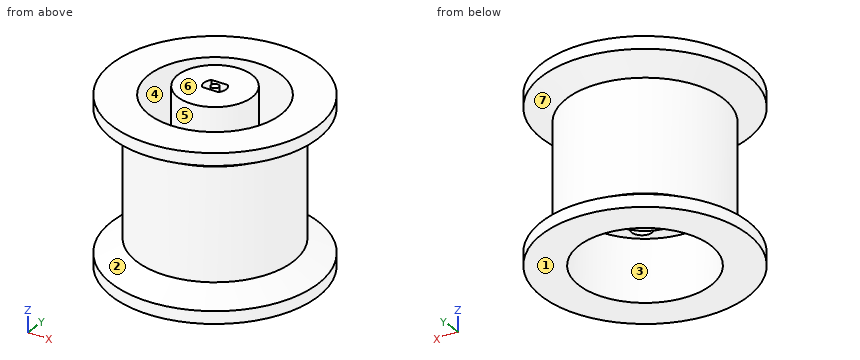
from build123d import *

# Parameters (mm, degrees)
ESQUISSE1_R                  = 25
ESQUISSE1_R_2                = 8
BOSS_EXTRU_1_DEPTH           = 20
ESQUISSE2_R                  = 16
ENL_V_MAT_EXTRU_1_DEPTH      = 15
ESQUISSE3_R                  = 2.5
ENL_V_MAT_EXTRU_2_DEPTH      = 44.301270189
R_P_TITION_CIRCULAIRE1_COUNT = 5
BOSS_EXTRU_2_DEPTH           = 17
BOSS_EXTRU_2_DEPTH_BACK      = 12
ESQUISSE4_R                  = 9
ESQUISSE4_R_2                = 8
BOSS_EXTRU_7_START           = -29
ESQUISSE13_R                 = 8
BOSS_EXTRU_7_DEPTH           = 29
ENL_V_MAT_EXTRU_3_DEPTH      = 7.7
ESQUISSE12_R                 = 0.945
BOSS_EXTRU_6_DEPTH           = 7.7


with BuildPart() as part:
    # Esquisse1 → Boss.-Extru.1 (new, symmetric)
    with BuildSketch(Plane.XY):
        Circle(ESQUISSE1_R)
        Circle(ESQUISSE1_R_2, mode=Mode.SUBTRACT)
    extrude(amount=BOSS_EXTRU_1_DEPTH, both=True)

    # Esquisse2 → Enlèv. mat.-Extru.1 (cut)
    with BuildSketch(Plane.XY.offset(20)):
        Circle(ESQUISSE2_R)
    enl_v_mat_extru_1 = extrude(amount=-ENL_V_MAT_EXTRU_1_DEPTH, mode=Mode.SUBTRACT)

    # Symétrie1: Enlèv. mat.-Extru.1 across plane
    add(enl_v_mat_extru_1.mirror(Plane.XY), mode=Mode.SUBTRACT)

    # Esquisse3 → Enlèv. mat.-Extru.2 (cut, through all)
    with BuildSketch(Plane.XY.offset(5)):
        with Locations((0, 12)):
            Circle(ESQUISSE3_R)
    enl_v_mat_extru_2 = extrude(amount=-ENL_V_MAT_EXTRU_2_DEPTH, mode=Mode.SUBTRACT)

    # Répétition circulaire1: Enlèv. mat.-Extru.2 ×5 about axis
    r_p_tition_circulaire1_axis = Axis((0, 0, 0), (0, 0, 1))
    for i in range(1, R_P_TITION_CIRCULAIRE1_COUNT):
        add(enl_v_mat_extru_2.rotate(r_p_tition_circulaire1_axis, i * 360 / R_P_TITION_CIRCULAIRE1_COUNT), mode=Mode.SUBTRACT)

    # Esquisse4 → Boss.-Extru.2 (add, two sides: drawn at the far end of the back side and taken through both)
    with BuildSketch(Plane.XY.offset(5).offset(-BOSS_EXTRU_2_DEPTH_BACK)):
        Circle(ESQUISSE4_R)
        Circle(ESQUISSE4_R_2, mode=Mode.SUBTRACT)
    extrude(amount=BOSS_EXTRU_2_DEPTH + BOSS_EXTRU_2_DEPTH_BACK)

    # Esquisse5 → Enlèvement de matière-Révolution1 (revolve, cut)
    with BuildSketch(Plane(origin=(0, 0, 0), x_dir=(1, 0, 0), z_dir=(0, 1, 0))):
        Polygon((-25, 17), (-19, 13.535898385), (-19, -13.535898385), (-25, -17), align=None)
    revolve(axis=Axis((0, 0, -25.284593115), (0, 0, 1)), mode=Mode.SUBTRACT)

    # Esquisse13 → Boss.-Extru.7 (add)
    with BuildSketch(Plane.XY.offset(22).offset(BOSS_EXTRU_7_START)):
        Circle(ESQUISSE13_R)
    extrude(amount=BOSS_EXTRU_7_DEPTH)

    # Esquisse11 → Enlèv. mat.-Extru.3 (cut)
    with BuildSketch(Plane.XY.offset(22)):
        with BuildLine():
            Line((-2.015, 1.8), (2.015, 1.8))
            ThreePointArc((2.015, 1.8), (2.695784465, 0), (2.015, -1.8))
            Line((2.015, -1.8), (-2.015, -1.8))
            ThreePointArc((-2.015, -1.8), (-2.695784465, 0), (-2.015, 1.8))
        make_face()
    extrude(amount=-ENL_V_MAT_EXTRU_3_DEPTH, mode=Mode.SUBTRACT)

    # Esquisse12 → Boss.-Extru.6 (add)
    with BuildSketch(Plane.XY.offset(14.3)):
        Circle(ESQUISSE12_R)
    extrude(amount=BOSS_EXTRU_6_DEPTH)


solid = part.part
For this review, take the finished solid that the model builds, in its own axes (mm). Face numbers are marked on the shaded views. A direction names the side the tool comes from. Round coordinates to 2 decimals unless told otherwise and drop trailing zeros. Write each loop counter-clockwise with the first axis right and the second up, starting at its lowest first coordinate (ties: lowest second). Pieces come first, ordered by that corner, then holes. Notation, with made-up numbers: M 49.25,70 L 68.25,70 A17 ccw 68.25,102 Z; hole C 1,37 d3. An arc over 180 degrees is marked long. Write item = value, one per line. Start each with the question number.
(1) For line 1 along Y through (x, z) = (0, 9); line 2 along Y through (x, z) = (0, -9.25); line 3 along Y through (x, z) = (1, -5.5), list the stretches that pass through material, from the lowest coordinate up.
(2) We need section A-A (z = 1.5). Give the boundary of the cut face in (x, y), then the cut area to 3 significant figures.
(3) For the marked faces 5, 6 and 7, list the 3-axis set-ups (+Z, -Z, +X, -X, +Y, -Y) from which the entire face can be reached by the end or side of a thin tool; tool diameter is ignored.
(4) The part is to be moulded in two halves that separate along Y. For the marked faces 1, 2, 3 and 4, say which applies: +Y half, -Y half, draft (parallel to the pull), parting line (faces both ways), or undercut.
(5) Clearance check with flat-ended pins moving along their axes: pin 1 Ø6 at (x, z) = (10.5, 0) entering from +Y; pin 2 Ø8 at (x, y) = (-13.5, -4.5) entering from +Z; pin 3 Ø9.5 at (x, y) = (3.5, -5) entering from -Z. State where each tip first meets the part, or that it passes through.
Results found:
q1.line_1 = -19 to -16, -9 to 9, 16 to 19
q1.line_2 = -19 to -16, 16 to 19
q1.line_3 = -18.97 to -15.97, -8.94 to 8.94, 15.97 to 18.97
q2.outline = C 0,0 d38; hole C -11.41,3.71 d5; hole C -7.05,-9.71 d5; hole C 0,12 d5; hole C 7.05,-9.71 d5; hole C 11.41,3.71 d5
q2.area = 1,040 mm²
q3.face_5 = +Z
q3.face_6 = +Z, +X, -X, +Y, -Y
q3.face_7 = none
q4.face_1 = draft
q4.face_2 = parting line
q4.face_3 = undercut
q4.face_4 = undercut
q5.pin_1 = 17.46
q5.pin_2 = 20
q5.pin_3 = -7
